Autodesk Inventor part; units mm, degrees
ref_plane "Work Plane2" through (-10.5, 431.6365, -532.8364) normal (0, 1, 0) x (1, 0, 0)
ref_plane "Work Plane3" through (0, 431.6365, -457.724) normal (0, 0, 1) x (1, 0, 0)
ref_plane "YZ Plane" through (0, 0, 0) normal (1, 0, 0) x (0, 1, 0)
sketch "profile" plane through (0, 0, 0) normal (0, 1, 0) x (-1, 0, 0)
  line L0 (12.5, 12.5) -> (-12.5, 12.5)
  line L1 (-12.5, 12.5) -> (-12.5, -12.5)
  line L2 (-12.5, -12.5) -> (12.5, -12.5)
  line L3 (12.5, -12.5) -> (12.5, 12.5)
  line L4 (-10, -10) -> (-10, 10)
  line L5 (-10, 10) -> (10, 10)
  line L6 (10, 10) -> (10, -10)
  line L7 (10, -10) -> (-10, -10)
  point P0 (0, 0)
  dimension "d0" = 12.5
  dimension "d1" = 25
  dimension "d2" = 25
  dimension "d3" = 12.5
  dimension "d6" = 2.5
sketch3d "3D Sketch1"
  line L0 (0, 0, 0) -> (0, 477.6365, -520.3364)
  dimension "d4" = 706.319
  dimension "d5" = 42.55
sweep "Sweep1" add profiles "profile" path "3D Sketch1"
fillet "Fillet1" radius 2 4 edges at (-12.5, 238.8182, -272.6682) (-12.5, 238.8182, -247.6682) (12.5, 238.8182, -247.6682) (12.5, 238.8182, -272.6682)
ref_plane "Work Plane2" through (-10.5, 431.6365, -532.8364) normal (0, 1, 0) x (1, 0, 0)
split "Split2" plane through (-10.5, 431.6365, -532.8364) removes the side toward (0, 1, 0)
ref_plane "Work Plane3" through (0, 431.6365, -457.724) normal (0, 0, 1) x (1, 0, 0)
split "Split3" plane through (0, 431.6365, -457.724) removes the side toward (0, 0, -1)
equation "\"d1\" = width"
equation "\"d2\" = d1"
equation "\"d6\" = t"
equation "\"d4\" = L"
equation "\"d5\" = angle"
equation "\"d9\" = filletRadius"
equation "\"L\" = 706.319"
equation "\"t\" = 2.5"
equation "\"filletRadius\" = 2"
equation "\"angle\" = 42.55deg"
equation "\"width\" = 25"
properties part number "support_truss2" material "Steel, Galvanized"
Verification items for the finished model (mm, model axes). A direction names the side the tool comes from. Coordinates: 2 decimals unless noted, no trailing zeros. Order: outer loops, then holes, each group sorted by start corner. A loop starts at its lowest first (then second) coordinate and runs counter-clockwise, first axis right, second up. Notation, with made-up numbers: M 70.25,55 L 124.25,55 A11 ccw 124.25,69 Z; hole C 41,9 d3. An arc over 180 degrees is marked long. Write each question's results on one line, items separated by ' | '.
1) Scan lines: line 1 along Y through (x, z) = (-0.5, -342.5); line 2 along Z through (x, y) = (8.75, 18.5); line 3 along Z through (x, y) = (5, 36). Record each from-to range of solid material in increasing order. Write a range as [from, to].
Solved:
line 1: y = [302.92, 305.21], [323.57, 325.87] | line 2: z = [-32.65, -30.15], [-10.15, -7.65] | line 3: z = [-51.72, -49.22], [-29.22, -26.72]
2) Release check for a two-part mould opening along X. For faces 1 (the face through (-10, 200, -223)), 2 (the face through (-12.5, 200, -225)), 3 (the face through (-0.147, 218.84, -225.904)) record: pulls with the +X half, pulls with the -X half, needs draft (parallel to the pull), parting line crosses it, or undercut.
Solved:
face 1: undercut | face 2: pulls with the -X half | face 3: needs draft
3) Section check A-A on x = 3.25. Record the cut outline in (y, z), plus the area to 3 significant figures.
Solved:
outline: M 0,-12.5 L 408.69,-457.72 L 410.98,-457.72 L 0,-10 Z; M 0,10 L 429.34,-457.72 L 431.64,-457.72 L 0,12.5 Z | area: 2,100 mm²
4) Access from +Z, -Z, +X, -X, +Y, -Y to the whole of each face (thin tool, end or side, straight path). Record for faces 4 (the face through (0, 0, -11)), 5 (the face through (0.14, 217.68, -227.14)).
Solved:
face 4: +Z, -Z, +X, -X, -Y | face 5: none
5) Gauge pin test, flat ends, axial feed: pin 1 Ø5 at (x, y) = (-3.5, 77) entering from -Z; pin 2 Ø3 at (x, z) = (4, -147.5) entering from +Y; pin 3 Ø1 at (x, z) = (-5, -186) entering from -Y. Record the tip position at first contact, or that the pin passes through.
Solved:
pin 1: stops at z = -99.11 | pin 2: stops at y = 148.25 | pin 3: stops at y = 158.8
